Print and shaded views of the part. All mm, measured from the part's lowest x, y and z. Round coordinates to 2 decimals unless told otherwise and drop trailing zeros. Write each loop counter-clockwise with the first axis right and the second up, starting at its lowest first coordinate (ties: lowest second). Pieces come first, ordered by that corner, then holes. Notation, with made-up numbers: M -2.5,13 L 8.5,13 A33 cw 8.5,41 Z; hole C -31.75,12 d6. An arc over 180 degrees is marked long. Write item = value, one per line. Start each with the question number.
Q1. Band-saw the part on C-C on z = 5.75. Write the cut outline in (x, y).
Q2. Band-saw the part on B-B on y = 18. Write the cut outline in (x, z).
Q3. Probe L1, parallel to Y at x = 39.75, z = 1.1; L2, parallel to Y at x = 6, z = 2.25; L3, parallel to Z at x = 20.5, y = 26. List the from-to ranges inside material, lowest first.
Q4. Drop flat-ended pins along their axis: P1, Ø1, axis at y = 3, z = 3, coming from the +X side; P2, Ø2.5, axis at x = 46.5, z = 2, coming from the -Y side; P3, Ø6, axis at x = 69.75, y = 18, coming from the +Z side. Give the stop position or say it passes through.
Q5. Band-saw the part on A-A on x = 39.75. Write the cut outline in (y, z).
Q6. Band-saw the part on D-D on z = 1.5. Write the cut outline in (x, y).
Q7. Pull direction X, two halves, no side cores. Call the marked faces 1 and 2: released by +X, released by -X, zero draft, split by the parting line, or undercut.
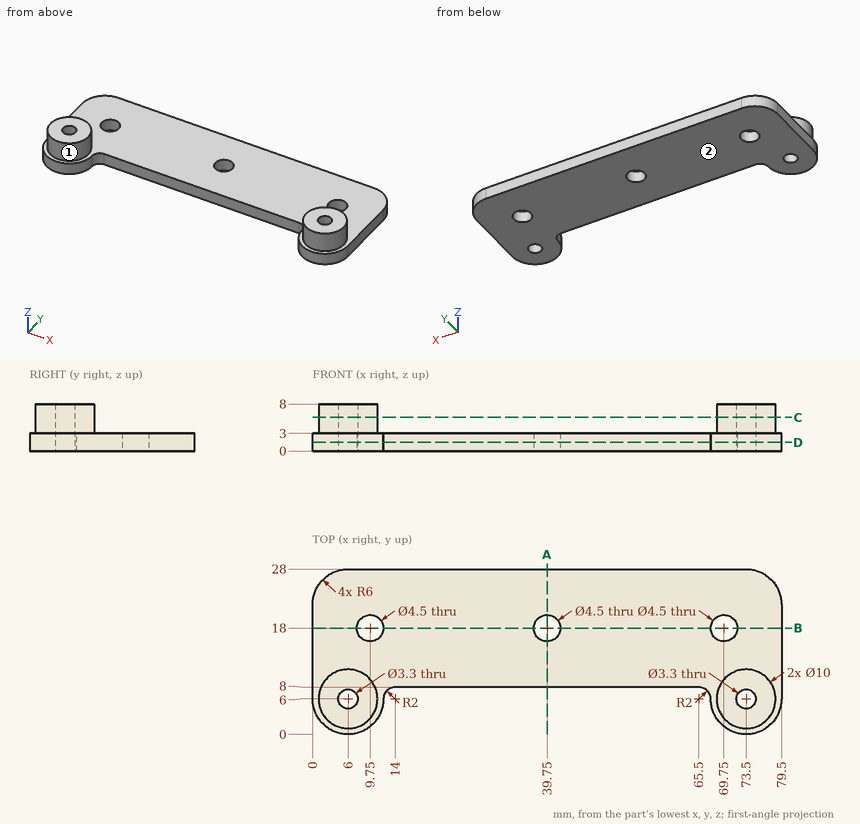
Conclusion:
q1.outline = C 6,6 d10; C 73.5,6 d10; hole C 6,6 d3.3; hole C 73.5,6 d3.3
q2.outline = M 0,0 L 7.5,0 L 7.5,3 L 0,3 Z; M 12,0 L 37.5,0 L 37.5,3 L 12,3 Z; M 42,0 L 67.5,0 L 67.5,3 L 42,3 Z; M 72,0 L 79.5,0 L 79.5,3 L 72,3 Z
q3.L1 = 8 to 15.75, 20.25 to 28
q3.L2 = 0 to 4.35, 7.65 to 28
q3.L3 = 0 to 3
q4.P1 = 78.95
q4.P2 = 8
q4.P3 = 3
q5.outline = M 8,0 L 15.75,0 L 15.75,3 L 8,3 Z; M 20.25,0 L 28,0 L 28,3 L 20.25,3 Z
q6.outline = M 0,6 A6 ccw 12,6 A2 cw 14,8 L 65.5,8 A2 cw 67.5,6 A6 ccw 79.5,6 L 79.5,22 A6 ccw 73.5,28 L 6,28 A6 ccw 0,22 Z; hole C 6,6 d3.3; hole C 9.75,18 d4.5; hole C 39.75,18 d4.5; hole C 69.75,18 d4.5; hole C 73.5,6 d3.3
q7.face_1 = undercut
q7.face_2 = zero draft
